Geometry: see drawing. Coordinates: mm, zero at the bounding-box minimum. A direction names the side the tool comes from. Coordinates: 2 decimals unless noted, no trailing zeros. Order: outer loops, then holes, each group sorted by start corner. A loop starts at its lowest first (then second) coordinate and runs counter-clockwise, first axis right, second up.
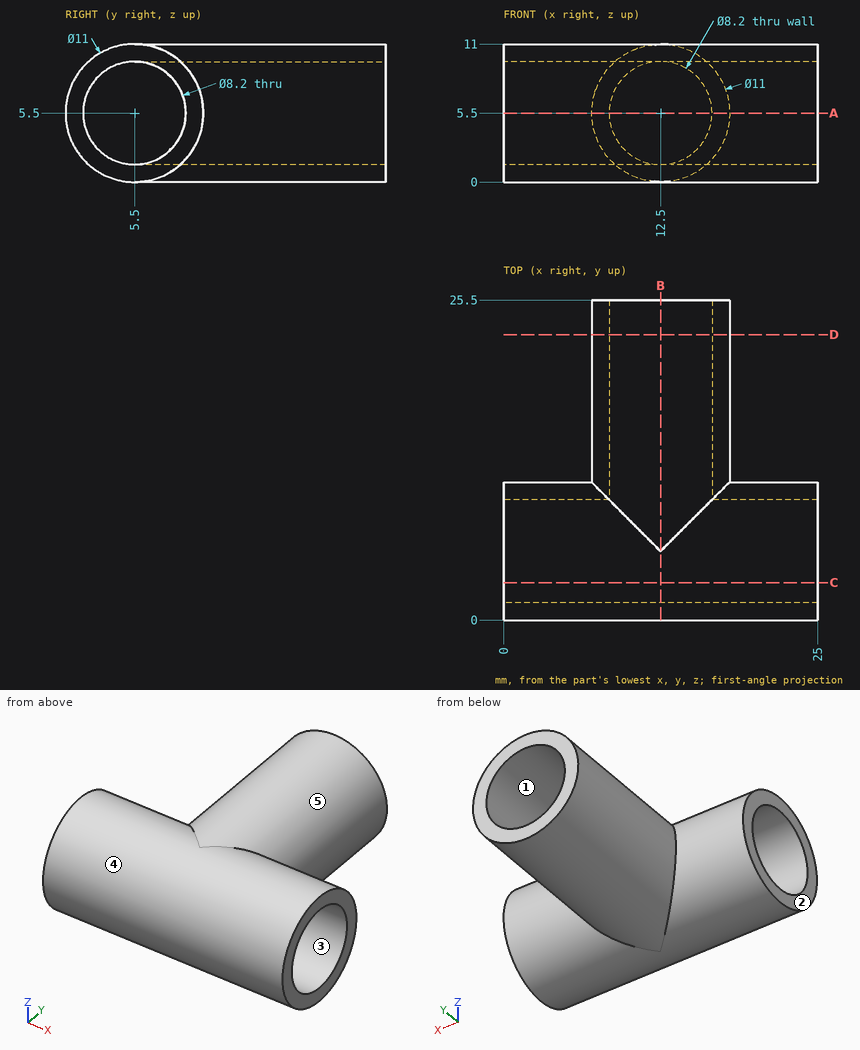
Item 1: Ray query, probe 1 along X at (y, z) = (17, 5.5); probe 2 along Y at (x, z) = (7.5, 5.5); probe 3 along Z at (x, y) = (13.25, 5.5). Return the intervals inside material, ascending.
Response values:
probe 1: x = 7 to 8.4, 16.6 to 18
probe 2: y = 0 to 1.4, 9.6 to 25.5
probe 3: z = 0 to 1.4, 9.6 to 11
Item 2: Cut plane D-D on y = 22.75. Return loops of the section in (x, z).
Response values:
outline: circle Ø11 at (12.5, 5.5); hole circle Ø8.2 at (12.5, 5.5)
Item 3: Cut plane B-B on x = 12.5. Return loops of the section in (y, z), then the cut area to 3 significant figures.
Response values:
outline: (5.5, 0) - (25.5, 0) - (25.5, 1.4) - (5.5, 1.4) arc R4.1 cw to (5.5, 9.6) - (25.5, 9.6) - (25.5, 11) - (5.5, 11) arc R5.5 ccw to start
area: 77.1 mm2
Item 4: Pin query (flat end, axial travel): pin 1 Ø1 at (x, z) = (20.5, 8.5) entering from +Y; pin 2 Ø5 at (y, z) = (17, 4) entering from +X; pin 3 Ø12 at (x, y) = (22, 13) entering from +Z. Return the tip coordinate at first contact, or that it passes through.
Response values:
pin 1: stops at y = 10.4
pin 2: stops at x = 18
pin 3: stops at z = 10.79
Item 5: Draft query along Y for the marked faces 3, 4 and 5. Return one class per face: pulls with the +Y half, pulls with the -Y half, needs draft (parallel to the pull), parting line crosses it, or undercut.
Response values:
face 3: undercut
face 4: parting line crosses it
face 5: needs draft
Item 6: Cut plane C-C on y = 3. Return loops of the section in (x, z), then the cut area to 3 significant figures.
Response values:
outline: (0, 0.6) - (25, 0.6) - (25, 2.25) - (0, 2.25) - close; (0, 8.75) - (25, 8.75) - (25, 10.4) - (0, 10.4) - close
area: 82.5 mm2
Item 7: Access query for the marked faces 1 and 2. Directions: +Z, -Z, +X, -X, +Y, -Y. A direction counts if a zero-diameter tool reaches every point of the face in a straight line with its end or side. Return the directions, or none.
Response values:
face 1: +Y
face 2: +Z, -Z, -X, +Y, -Y
Item 8: Cut plane A-A on z = 5.5. Return loops of the section in (x, y).
Response values:
outline: (0, 0) - (25, 0) - (25, 1.4) - (0, 1.4) - close; (0, 9.6) - (8.4, 9.6) - (8.4, 25.5) - (7, 25.5) - (7, 11) - (0, 11) - close; (16.6, 9.6) - (25, 9.6) - (25, 11) - (18, 11) - (18, 25.5) - (16.6, 25.5) - close
